CAD build for the part. Positions are in the model's coordinates, mm. A direction names the side the tool comes from. Round coordinates to 2 decimals unless told otherwise and drop trailing zeros. Order: outer loops, then holes, each group sorted by start corner. A loop starts at its lowest first (then second) coordinate and runs counter-clockwise, first axis right, second up. Notation, with made-up numbers: M 57,0 L 115,0 A20 cw 115,13 Z; hole C -28,-12 d9. An arc over 180 degrees is marked long. Put each result on its own line as item: value.
```python
from build123d import *

# Parameters (mm, degrees)
SKETCH1_W           = 100
SKETCH1_H           = 30
BOSS_EXTRUDE1_DEPTH = 5
SKETCH2_R           = 15
BOSS_EXTRUDE2_DEPTH = 3
CUT_EXTRUDE1_DEPTH  = 9
SKETCH4_R           = 3
CUT_EXTRUDE2_DEPTH  = 6
CHAMFER1_SIZE       = 8
CHAMFER1_SIZE2      = 45
CHAMFER2_SIZE       = 45
CHAMFER2_SIZE2      = 8
CHAMFER3_SIZE       = 45
CHAMFER3_SIZE2      = 8
CHAMFER4_SIZE       = 8
CHAMFER4_SIZE2      = 45
FILLET1_R           = 8
CUT_EXTRUDE3_DEPTH  = 6
FILLET2_R           = 30
CUT_EXTRUDE4_DEPTH  = 3
FILLET3_R           = 0.5


with BuildPart() as part:
    # Sketch1 → Boss-Extrude1 (new body)
    with BuildSketch(Plane(origin=(0, 0, 0), x_dir=(1, 0, 0), z_dir=(0, 1, 0))):
        Rectangle(SKETCH1_W, SKETCH1_H)
    extrude(amount=BOSS_EXTRUDE1_DEPTH)

    # Sketch2 → Boss-Extrude2 (add)
    with BuildSketch(Plane(origin=(0, 5, 0), x_dir=(1, 0, 0), z_dir=(0, 1, 0))):
        Circle(SKETCH2_R)
    extrude(amount=BOSS_EXTRUDE2_DEPTH)

    # Sketch3 → Cut-Extrude1 (cut, through all)
    with BuildSketch(Plane(origin=(0, 8, 0), x_dir=(1, 0, 0), z_dir=(0, 1, 0))):
        with BuildLine():
            Line((-2, 6.5), (-2, 8.5))
            ThreePointArc((-2, 8.5), (0, 10.5), (2, 8.5))
            Line((2, 8.5), (2, 6.5))
            ThreePointArc((2, 6.5), (0, 4.5), (-2, 6.5))
        make_face()
        with BuildLine():
            Line((-2, -8.5), (-2, -6.5))
            ThreePointArc((-2, -6.5), (0, -4.5), (2, -6.5))
            Line((2, -6.5), (2, -8.5))
            ThreePointArc((2, -8.5), (0, -10.5), (-2, -8.5))
        make_face()
    extrude(amount=-CUT_EXTRUDE1_DEPTH, mode=Mode.SUBTRACT)

    # Sketch4 → Cut-Extrude2 (cut, through all)
    with BuildSketch(Plane(origin=(0, 5, 0), x_dir=(1, 0, 0), z_dir=(0, 1, 0))):
        with Locations((40, 0)):
            Circle(SKETCH4_R)
        with Locations((-40, 0)):
            Circle(SKETCH4_R)
    extrude(amount=-CUT_EXTRUDE2_DEPTH, mode=Mode.SUBTRACT)

    # Chamfer1
    chamfer1_edges = [part.edges().sort_by_distance(p)[0] for p in [
        (50, 2.5, -15),
    ]]
    chamfer1_side = [part.faces().sort_by_distance(p)[0] for p in [
        (50, 2.5, 0),
    ]]
    chamfer(chamfer1_edges, length=CHAMFER1_SIZE, length2=CHAMFER1_SIZE2, reference=chamfer1_side[0])

    # Chamfer2
    chamfer2_edges = [part.edges().sort_by_distance(p)[0] for p in [
        (50, 2.5, 15),
    ]]
    chamfer2_side = [part.faces().sort_by_distance(p)[0] for p in [
        (0, 2.5, 15),
    ]]
    chamfer(chamfer2_edges, length=CHAMFER2_SIZE, length2=CHAMFER2_SIZE2, reference=chamfer2_side[0])

    # Chamfer3
    chamfer3_edges = [part.edges().sort_by_distance(p)[0] for p in [
        (-50, 2.5, -15),
    ]]
    chamfer3_side = [part.faces().sort_by_distance(p)[0] for p in [
        (-22.5, 2.5, -15),
    ]]
    chamfer(chamfer3_edges, length=CHAMFER3_SIZE, length2=CHAMFER3_SIZE2, reference=chamfer3_side[0])

    # Chamfer4
    chamfer4_edges = [part.edges().sort_by_distance(p)[0] for p in [
        (-50, 2.5, 15),
    ]]
    chamfer4_side = [part.faces().sort_by_distance(p)[0] for p in [
        (-50, 2.5, 4),
    ]]
    chamfer(chamfer4_edges, length=CHAMFER4_SIZE, length2=CHAMFER4_SIZE2, reference=chamfer4_side[0])

    # Fillet1
    fillet1_edges = [part.edges().sort_by_distance(p)[0] for p in [
        (50, 2.5, -7),
        (50, 2.5, 7),
        (-50, 2.5, -7),
        (-50, 2.5, 7),
    ]]
    fillet(fillet1_edges, radius=FILLET1_R)

    # Sketch5 → Cut-Extrude3 (cut, through all)
    with BuildSketch(Plane(origin=(0, 5, 0), x_dir=(1, 0, 0), z_dir=(0, 1, 0))):
        with BuildLine():
            Line((-16.487122597, 8.895126691), (-33.221241877, 5.920172153))
            ThreePointArc((-33.221241877, 5.920172153), (-31, 0), (-33.221241877, -5.920172153))
            Line((-33.221241877, -5.920172153), (-16.487122597, -8.895126691))
            ThreePointArc((-16.487122597, -8.895126691), (-19, 0), (-16.487122597, 8.895126691))
        make_face()
    cut_extrude3 = extrude(amount=-CUT_EXTRUDE3_DEPTH, mode=Mode.SUBTRACT)

    # Mirror2: Cut-Extrude3 across plane
    add(cut_extrude3.mirror(Plane(origin=(0, 0, 0), x_dir=(0, 0, 1), z_dir=(1, 0, 0))), mode=Mode.SUBTRACT)

    # Fillet2
    fillet2_edges = [part.edges().sort_by_distance(p)[0] for p in [
        (5, 2.5, -15),
        (5, 2.5, 15),
        (-5, 2.5, -15),
        (-5, 2.5, 15),
    ]]
    fillet(fillet2_edges, radius=FILLET2_R)

    # Sketch7 → Cut-Extrude4 (cut)
    with BuildSketch(Plane.XZ):
        with BuildLine():
            Line((-4, 8.5), (-4, 6.5))
            ThreePointArc((-4, 6.5), (0, 2.5), (4, 6.5))
            Line((4, 6.5), (4, 8.5))
            ThreePointArc((4, 8.5), (0, 12.5), (-4, 8.5))
        make_face()
    cut_extrude4 = extrude(amount=-CUT_EXTRUDE4_DEPTH, mode=Mode.SUBTRACT)

    # Mirror3: Cut-Extrude4 across plane
    add(cut_extrude4.mirror(Plane.XY), mode=Mode.SUBTRACT)

    # Fillet3
    fillet3_edges = [part.edges().sort_by_distance(p)[0] for p in [
        (0, 0, 12.5),
        (-4, 0, 7.5),
        (0, 0, 2.5),
        (4, 0, 7.5),
        (0, 0, -12.5),
        (-4, 0, -7.5),
        (0, 0, -2.5),
        (4, 0, -7.5),
    ]]
    fillet(fillet3_edges, radius=FILLET3_R)


solid = part.part
```
Item 1: Band-saw the part on C-C on x = 40. Give the cut face in (y, z), and give its area (3 significant figures).
Answers below:
outline: M 0,-8.78 L 5,-8.78 L 5,-3 L 0,-3 Z; M 0,3 L 5,3 L 5,8.78 L 0,8.78 Z
area: 57.8 mm²
Item 2: Band-saw the part on A-A on y = 4. State how many separate pieces and enclosed holes the cut face has, and give its area (3 significant figures).
Answers below:
separate pieces: 1
enclosed holes: 6
area: 1,750 mm²
Item 3: Band-saw the part on B-B on x = 26.5. Give the cut face in (y, z), and give its area (3 significant figures).
Answers below:
outline: M 0,-11.18 L 5,-11.18 L 5,-7.12 L 0,-7.12 Z; M 0,7.12 L 5,7.12 L 5,11.18 L 0,11.18 Z
area: 40.6 mm²
Item 4: Probe line 1 along X through (y, z) = (3.6, 0); line 2 along X through (y, z) = (3.5, -5.5); line 3 along Y through (x, z) = (-31, -9.25). List the from-to ranges inside material, lowest first. Write a range as [from, to].
Answers below:
line 1: [-50, -43], [-37, -31], [-19, 19], [31, 37], [43, 50]
line 2: [-48.08, -32.88], [-18.09, -1.73], [1.73, 18.09], [32.88, 48.08]
line 3: [0, 5]
Item 5: Mould opens along X. For faces 4 (the cylindrical face through (-48.182, 2.535, 5.375)), 5 (the flat face through (2, 6, -8)), 6 (the cylindrical face through (-14.985, 6.479, -0.66)) say: pulls with the +X half, pulls with the -X half, needs draft (parallel to the pull), parting line crosses it, or undercut.
Answers below:
face 4: pulls with the -X half
face 5: undercut
face 6: parting line crosses it
Item 6: Pin check, flat tips, straight feed: P1, Ø9.5, axis at x = 40, z = 0, coming from the +Y side; P2, Ø1, axis at y = 1.5, z = 3.5, coming from the +X side; P3, Ø1, axis at y = 2, z = -7, coming from the -X side. Stop position of each tip, or through.
Answers below:
P1: y = 5
P2: x = 49.53
P3: x = -47.05
Item 7: Tool access for faces 1 (the flat face through (4, 2, 7)), 2 (the flat face through (-24.737, 2.535, -7.428)), 3 (the cylindrical face through (4.953, 2.535, 14.887)): list every direction of +Z, -Z, +X, -X, +Y, -Y with a clear straight run to the whole face (end or side of a thin tool).
Answers below:
face 1: -Y
face 2: +Y, -Y
face 3: +Z, +X, +Y, -Y
